Can you work these out from the model? Positions are in its coordinate system, mm. A direction names the side the tool comes from. Round coordinates to 2 decimals unless told otherwise and drop trailing zeros. Loops run counter-clockwise (first coordinate to the right, second up) from the corner with the lowest first, then second, coordinate; pieces in that order, holes last. Notation, with made-up numbers: (-37, 72) -> (9, 72) arc R12 cw to (9, 92) -> close; hole circle Ø9 at (89.25, 28). An arc over 180 degrees is marked (long way). Answer as a JSON object with one key per item and string values.
```python
from build123d import *

# Parameters (mm, degrees)
SKETCH1_W           = 10
SKETCH1_H           = 15
BOSS_EXTRUDE1_DEPTH = 15
SKETCH3_W           = 5
SKETCH3_H           = 2.3
BOSS_EXTRUDE2_DEPTH = 15
SKETCH4_R           = 3.315
CUT_EXTRUDE1_DEPTH  = 24.452078799
SKETCH6_W           = 2
SKETCH6_H           = 15
CUT_EXTRUDE2_DEPTH  = 8
BOSS_EXTRUDE3_DEPTH = 5


with BuildPart() as part:
    # Sketch1 → Boss-Extrude1 (new body)
    with BuildSketch(Plane.XY):
        Rectangle(SKETCH1_W, SKETCH1_H)
    extrude(amount=BOSS_EXTRUDE1_DEPTH)

    # Sketch3 → Boss-Extrude2 (add)
    with BuildSketch(Plane.XY.offset(15)):
        with Locations((-7.5, -6.35)):
            Rectangle(SKETCH3_W, SKETCH3_H)
        with Locations((7.5, -6.35)):
            Rectangle(SKETCH3_W, SKETCH3_H)
    extrude(amount=-BOSS_EXTRUDE2_DEPTH)

    # Sketch4 → Cut-Extrude1 (cut, through all)
    with BuildSketch(Plane.XZ.offset(7.5)):
        with Locations(Location((0, 7.5, 0), (0, 0, 270))):
            Circle(SKETCH4_R)
    extrude(amount=-CUT_EXTRUDE1_DEPTH, mode=Mode.SUBTRACT)

    # Sketch6 → Cut-Extrude2 (cut)
    with BuildSketch(Plane.XY.offset(15)):
        Rectangle(SKETCH6_W, SKETCH6_H)
    extrude(amount=-CUT_EXTRUDE2_DEPTH, mode=Mode.SUBTRACT)

    # Sketch7 → Boss-Extrude3 (add)
    with BuildSketch(Plane.XZ.offset(7.5)):
        with BuildLine():
            Line((3, 15), (10, 15))
            Line((10, 15), (10, 0))
            Line((10, 0), (-10, 0))
            Line((-10, 0), (-10, 15))
            Line((-10, 15), (-3, 15))
            Line((-3, 15), (-3, 11.887393873))
            ThreePointArc((-3, 11.887393873), (0, 2.185), (3, 11.887393873))
            Line((3, 11.887393873), (3, 15))
        make_face()
    extrude(amount=BOSS_EXTRUDE3_DEPTH)


solid = part.part
```
Q1. I want a section at A-A, the plane z = 7.5. Write out the boundary of the cut face in (x, y) (3 decimals).
Determined:
{"outline": "(-10, -12.5) -> (-5.315, -12.5) -> (-5.315, -7.5) -> (-3.315, -7.5) -> (-3.315, 7.5) -> (-5, 7.5) -> (-5, -5.2) -> (-10, -5.2) -> close; (3.315, -7.5) -> (5.315, -7.5) -> (5.315, -12.5) -> (10, -12.5) -> (10, -5.2) -> (5, -5.2) -> (5, 7.5) -> (3.315, 7.5) -> close"}
Q2. If I drill on L1, parallel to X at y = -4.75, z = 12; L2, parallel to X at y = -9.35, z = 7.5 (3 decimals); L3, parallel to Y at x = -7, z = 6, over which ranges is the centre line in solid material (lowest first)? Write a range as [from, to].
Determined:
{"L1": "[-5, -1], [1, 5]", "L2": "[-10, -5.315], [5.315, 10]", "L3": "[-12.5, -5.2]"}
Q3. I want a section at C-C, the plane x = 1.5. Write out the boundary of the cut face in (y, z), then the cut area to 3 significant figures.
Determined:
{"outline": "(-12.5, 0) -> (7.5, 0) -> (7.5, 4.54) -> (-7.5, 4.54) -> (-7.5, 2.4) -> (-12.5, 2.4) -> close; (-7.5, 10.46) -> (7.5, 10.46) -> (7.5, 15) -> (-7.5, 15) -> close", "area": "148 mm²"}
Q4. I want a section at D-D, the plane z = 5.25. Write out the boundary of the cut face in (x, y).
Determined:
{"outline": "(-10, -12.5) -> (-4.82, -12.5) -> (-4.82, -7.5) -> (-2.43, -7.5) -> (-2.43, 7.5) -> (-5, 7.5) -> (-5, -5.2) -> (-10, -5.2) -> close; (2.43, -7.5) -> (4.82, -7.5) -> (4.82, -12.5) -> (10, -12.5) -> (10, -5.2) -> (5, -5.2) -> (5, 7.5) -> (2.43, 7.5) -> close"}
Q5. I want a section at B-B, the plane y = -6.75. Write out the boundary of the cut face in (x, z) (3 decimals).
Determined:
{"outline": "(-10, 0) -> (10, 0) -> (10, 15) -> (1, 15) -> (1, 10.661) arc R3.315 cw (long way) to (-1, 10.661) -> (-1, 15) -> (-10, 15) -> close"}
Q6. I'm going to push flat-ended pins straight in: pin 1 (2 mm diameter, centred on x = -2.5, z = 7.5, fed in from -Y); pin 2 (1.5 mm diameter, centred on x = 7, y = 5, fed in from -Z); pin 3 (8 mm diameter, centred on x = 7.5, y = 1.5, fed in from +Z); pin 4 (4 mm diameter, centred on x = 8.5, z = 9.5, fed in from +Y). Where does each tip first touch, or does it pass through?
Determined:
{"pin 1": "y = -7.5", "pin 2": "through", "pin 3": "z = 15", "pin 4": "y = -5.2"}
Q7. We'd pull the mould along Z, two halves only. Please class faces 1 (the flat face through (-5, 1, 7)), 2 (the cylindrical face through (-0.132, -0.105, 4.188)), 3 (the flat face through (-2.4, -7.5, 10.1)), 4 (the flat face through (4, -5, 15)): pulls with the +Z half, pulls with the -Z half, needs draft (parallel to the pull), parting line crosses it, or undercut.
Determined:
{"face 1": "needs draft", "face 2": "undercut", "face 3": "undercut", "face 4": "pulls with the +Z half"}
Q8. On a 3-axis mill with a long thin cutter (end or side, diameter ignored), from which of +Z, -Z, +X, -X, +Y, -Y can I reach the whole of each face in a straight line? I mean faces 5 (the flat face through (5, 1, 7)), 6 (the flat face through (1, 0, 13)), 7 (the cylindrical face through (-0.19, -9.96, 2.19)), 8 (the flat face through (-3, -10, 13)). Say none if no direction works.
Determined:
{"face 5": "+Z, -Z, +X, +Y", "face 6": "+Z, +Y, -Y", "face 7": "-Y", "face 8": "+Z, -Y"}
